```python
from build123d import *

# Parameters (mm, degrees)
SKETCH3_R   = 1.5
SKETCH3_W   = 14
SKETCH3_H   = 14
LASER_DEPTH = 3


with BuildPart() as part:
    # Sketch3 → Laser (new body)
    with BuildSketch(Plane(origin=(0, 0, 0), x_dir=(1, 0, 0), z_dir=(0, 1, 0))):
        with BuildLine():
            Line((-14.486734177, 37), (157, 37))
            ThreePointArc((157, 37), (159.121320344, 36.121320344), (160, 34))
            Line((160, 34), (160, -80.984375239))
            ThreePointArc((160, -80.984375239), (159.129622744, -83.097360561), (157.023528688, -83.984282971))
            Line((157.023528688, -83.984282971), (27.26862569, -85.001968485))
            ThreePointArc((27.26862569, -85.001968485), (-2.456705292, -92.729196832), (-24.985922812, -113.603576292))
            ThreePointArc((-24.985922812, -113.603576292), (-27.026813158, -114.929395936), (-29.379241112, -114.305606027))
            Line((-29.379241112, -114.305606027), (-52.510135606, -95.72030429))
            ThreePointArc((-52.510135606, -95.72030429), (-58.054538693, -89.41838891), (-61.142600429, -81.61336375))
            ThreePointArc((-61.142600429, -81.61336375), (-63.620659677, -72.842256523), (-67.314962408, -64.51007632))
            Line((-67.314962408, -64.51007632), (-97.34041061, -7.990411949))
            ThreePointArc((-97.34041061, -7.990411949), (-97.559643654, -5.704801569), (-96.098494227, -3.933609797))
            Line((-96.098494227, -3.933609797), (-23.071235452, 34.86131583))
            ThreePointArc((-23.071235452, 34.86131583), (-18.910183965, 36.457280449), (-14.486734177, 37))
        make_face()
        with Locations(Location((-22.393572022, 24.996840478, 0), (0, 0, 270))):
            Circle(SKETCH3_R, mode=Mode.SUBTRACT)
        with Locations(Location((-6.470173498, -4.977237981, 0), (0, 0, 270))):
            Circle(SKETCH3_R, mode=Mode.SUBTRACT)
        with Locations(Location((-36.444251957, -20.900636504, 0), (0, 0, 270))):
            Circle(SKETCH3_R, mode=Mode.SUBTRACT)
        with Locations(Location((-52.367650481, 9.073441955, 0), (0, 0, 270))):
            Circle(SKETCH3_R, mode=Mode.SUBTRACT)
        with Locations((9, -10)):
            Rectangle(SKETCH3_W, SKETCH3_H, mode=Mode.SUBTRACT)
        with Locations((9, 9)):
            Rectangle(SKETCH3_W, SKETCH3_H, mode=Mode.SUBTRACT)
        with Locations((28, 11)):
            Rectangle(SKETCH3_W, SKETCH3_H, mode=Mode.SUBTRACT)
        with Locations((47, 23)):
            Rectangle(SKETCH3_W, SKETCH3_H, mode=Mode.SUBTRACT)
        with Locations((66, 18)):
            Rectangle(SKETCH3_W, SKETCH3_H, mode=Mode.SUBTRACT)
        with Locations((85, 9)):
            Rectangle(SKETCH3_W, SKETCH3_H, mode=Mode.SUBTRACT)
        with Locations((104, 6)):
            Rectangle(SKETCH3_W, SKETCH3_H, mode=Mode.SUBTRACT)
        with Locations((123, 6)):
            Rectangle(SKETCH3_W, SKETCH3_H, mode=Mode.SUBTRACT)
        with Locations((146, 1.25)):
            Rectangle(SKETCH3_W, SKETCH3_H, mode=Mode.SUBTRACT)
        with Locations((146, -65.25)):
            Rectangle(SKETCH3_W, SKETCH3_H, mode=Mode.SUBTRACT)
        with Locations((28, -8)):
            Rectangle(SKETCH3_W, SKETCH3_H, mode=Mode.SUBTRACT)
        with Locations((47, 4)):
            Rectangle(SKETCH3_W, SKETCH3_H, mode=Mode.SUBTRACT)
        with Locations((66, -1)):
            Rectangle(SKETCH3_W, SKETCH3_H, mode=Mode.SUBTRACT)
        with Locations((85, -10)):
            Rectangle(SKETCH3_W, SKETCH3_H, mode=Mode.SUBTRACT)
        with Locations((104, -13)):
            Rectangle(SKETCH3_W, SKETCH3_H, mode=Mode.SUBTRACT)
        with Locations((123, -13)):
            Rectangle(SKETCH3_W, SKETCH3_H, mode=Mode.SUBTRACT)
        with Locations((9, -29)):
            Rectangle(SKETCH3_W, SKETCH3_H, mode=Mode.SUBTRACT)
        with Locations((28, -27)):
            Rectangle(SKETCH3_W, SKETCH3_H, mode=Mode.SUBTRACT)
        with Locations((47, -15)):
            Rectangle(SKETCH3_W, SKETCH3_H, mode=Mode.SUBTRACT)
        with Locations((66, -20)):
            Rectangle(SKETCH3_W, SKETCH3_H, mode=Mode.SUBTRACT)
        with Locations((85, -29)):
            Rectangle(SKETCH3_W, SKETCH3_H, mode=Mode.SUBTRACT)
        with Locations((104, -32)):
            Rectangle(SKETCH3_W, SKETCH3_H, mode=Mode.SUBTRACT)
        with Locations((123, -32)):
            Rectangle(SKETCH3_W, SKETCH3_H, mode=Mode.SUBTRACT)
        with Locations((9, -48)):
            Rectangle(SKETCH3_W, SKETCH3_H, mode=Mode.SUBTRACT)
        with Locations((28, -46)):
            Rectangle(SKETCH3_W, SKETCH3_H, mode=Mode.SUBTRACT)
        with Locations((47, -34)):
            Rectangle(SKETCH3_W, SKETCH3_H, mode=Mode.SUBTRACT)
        with Locations((66, -39)):
            Rectangle(SKETCH3_W, SKETCH3_H, mode=Mode.SUBTRACT)
        with Locations((85, -48)):
            Rectangle(SKETCH3_W, SKETCH3_H, mode=Mode.SUBTRACT)
        Polygon((-86.936243665, -12.654456356), (-74.572567085, -6.086389562), (-68.004500291, -18.450066143), (-80.368176871, -25.018132937), align=None, mode=Mode.SUBTRACT)
        with Locations((13.75, -71)):
            Rectangle(SKETCH3_W, SKETCH3_H, mode=Mode.SUBTRACT)
        with Locations((108.75, -51)):
            Rectangle(SKETCH3_W, SKETCH3_H, mode=Mode.SUBTRACT)
        with Locations((108.75, -70)):
            Rectangle(SKETCH3_W, SKETCH3_H, mode=Mode.SUBTRACT)
        Polygon((-65.65876215, -22.865664922), (-78.022438731, -29.433731716), (-71.454371937, -41.797408296), (-59.090695356, -35.229341502), align=None, mode=Mode.SUBTRACT)
        Polygon((-52.329358437, -37.29920214), (-39.965681856, -30.731135346), (-33.397615062, -43.094811927), (-45.761291642, -49.662878721), align=None, mode=Mode.SUBTRACT)
        Polygon((-26.636278142, -45.164672565), (-14.272601562, -38.596605771), (-7.704534768, -50.960282351), (-20.068211348, -57.528349145), align=None, mode=Mode.SUBTRACT)
        Polygon((-31.051876921, -47.510410705), (-43.415553502, -54.078477499), (-36.847486708, -66.44215408), (-24.483810127, -59.874087286), align=None, mode=Mode.SUBTRACT)
        Polygon((-47.831152281, -56.42421564), (-60.194828861, -62.992282434), (-53.626762067, -75.355959015), (-41.263085486, -68.787892221), align=None, mode=Mode.SUBTRACT)
        Polygon((-34.094882695, -83.577777362), (-42.863777875, -94.491368765), (-31.950186473, -103.260263946), (-23.181291292, -92.346672543), align=None, mode=Mode.SUBTRACT)
        Polygon((-23.864729376, -75.115009761), (-11.501052796, -68.546942967), (-4.932986002, -80.910619548), (-17.296662582, -87.478686342), align=None, mode=Mode.SUBTRACT)
        Polygon((-38.884783677, 4.94590688), (-26.521107096, 11.513973674), (-19.953040302, -0.849702906), (-32.316716883, -7.4177697), align=None, mode=Mode.SUBTRACT)
    extrude(amount=-LASER_DEPTH)


solid = part.part
```
The listing builds one solid part. Answer for the finished solid, in the listing's coordinates (mm). A direction names the side the tool comes from. Coordinates: 2 decimals unless noted, no trailing zeros. Use one line per item in the form item = value. Start each with the question number.
Item 1: A tool of negligible diameter and unlimited length cuts with its end or side. For faces 3 (the face through (-82.118, -1.479, 36.646)), 4 (the face through (-27.627, -1.479, 97.88)), from which of +Z, -Z, +X, -X, +Y, -Y can it reach the whole face along a straight path? Write none if from no direction.
Item 2: The mould has two halves that part along X. Classify faces 1 (the face through (-57.99, -1.48, 89.52)), 2 (the face through (-37.5, -1.5, 98.8)): released by +X, released by -X, zero draft, split by the parting line, or undercut.
Item 3: Consider L1, parallel to Z at x = 29.5, y = -1.2; L2, parallel to Z at x = 141, y = -1.25; L3, parallel to Z at x = -51, y = -1.05. Determine where each line is inside the solid, lowest interval first. Write a range as [from, to].
Item 4: The part is cut by section A-A on y = -2.15. Count the separate pieces of the cut face and the enclosed holes in it, then the cut area to 3 significant figures.
Item 5: Flat-ended cylindrical pins translate along their axes: pin 1 Ø0.9 at (y, z) = (-1.5, 20) entering from -X; pin 2 Ø0.9 at (y, z) = (-1, 16) entering from -X; pin 3 Ø0.9 at (y, z) = (-1.5, 11.5) entering from -X. Find the tip coordinate at first contact, or state that the pin passes through.
Answer key:
q1.face_3 = +Z, -X, +Y, -Y
q1.face_4 = +Y, -Y
q2.face_1 = released by -X
q2.face_2 = undercut
q3.L1 = [-37, -18], [-4, 1], [15, 20], [34, 39], [53, 84.98]
q3.L2 = [-37, -8.25], [5.75, 58.25], [72.25, 84.11]
q3.L3 = [-20.02, -9.69], [-8.46, 36.59], [39.8, 58.11], [73.96, 96.93]
q4.separate_pieces = 1
q4.enclosed_holes = 44
q4.area = 21,400 mm2
q5.pin_1 = -91.2
q5.pin_2 = -93.32
q5.pin_3 = -95.72
